Could you check a few things on this model? Use its own coordinates, in mm. A direction names the side the tool comes from. Give positions to 0.01 mm unless a question says otherwise; leave off trailing zeros. Loops run counter-clockwise (first coordinate to the right, second up) from the corner with the lowest first, then second, coordinate; pieces in that order, holes last. Notation, with made-up numbers: (25, -16) -> (37, -16) arc R23 ccw to (37, 18) -> close; hole circle Ø11 at (65.25, 45.25). An arc over 180 degrees is marked (long way). Put each result on its own line as item: value.
```python
from build123d import *

# Parameters (mm, degrees)
F0_R     = 11
F1_DEPTH = 3
F3_DEPTH = 3
F4_R     = 1
F5_DEPTH = 1


with BuildPart() as f1:
    # F0 (on Top) → F1 (new body)
    with BuildSketch(Plane.XY):
        Circle(F0_R)
    extrude(amount=F1_DEPTH)

    # F2 (on face) → F3 (cut)
    with BuildSketch(Plane.XY.offset(3)):
        with BuildLine():
            ThreePointArc((1.140175, -1.05), (0, 1.55), (-1.140175, -1.05))
            Line((-1.140175, -1.05), (1.140175, -1.05))
        make_face()
    extrude(amount=-F3_DEPTH, mode=Mode.SUBTRACT)

    # F4 (on face) → F5 (cut)
    with BuildSketch(Plane.XY.offset(3)):
        with Locations((-1.606246, 9.109472)):
            Circle(F4_R)
        with Locations((-7.085911, -5.945785)):
            Circle(F4_R)
        with Locations((1.606246, 9.109472)):
            Circle(F4_R)
        with Locations((-8.692157, -3.163686)):
            Circle(F4_R)
        with Locations((8.692157, -3.163686)):
            Circle(F4_R)
        with Locations((7.085911, -5.945785)):
            Circle(F4_R)
    extrude(amount=-F5_DEPTH, mode=Mode.SUBTRACT)


solid = f1.part
```
1. If we section it at D-D (y = 9.75): List the corners of the cut face in (x, z) for me, then the cut area to 3 significant figures.
Recorded:
outline: (-5.09, 0) -> (5.09, 0) -> (5.09, 3) -> (2.37, 3) -> (2.37, 2) -> (0.84, 2) -> (0.84, 3) -> (-0.84, 3) -> (-0.84, 2) -> (-2.37, 2) -> (-2.37, 3) -> (-5.09, 3) -> close
area: 27.5 mm^2
2. For faces 1 (the face through (0, -2, 0)), 2 (the face through (0, -1.05, 2)), 3 (the face through (-1.74, 10.1, 2.51)), which set-ups out of +Z, -Z, +X, -X, +Y, -Y let a thin tool reach every point of the face, with its end or its side?
Recorded:
face 1: -Z, +X, -X, +Y, -Y
face 2: +Z, -Z
face 3: +Z
3. I'm going to push flat-ended pins straight in: pin 1 (2 mm diameter, centred on x = -9, y = -3, fed in from +Z); pin 2 (1 mm diameter, centred on x = -8, z = 2.5, fed in from -Y); pin 3 (1.2 mm diameter, centred on x = -7.09, y = -5.95, fed in from +Z). Where does each tip first touch, or does it pass through?
Recorded:
pin 1: stops at z = 3
pin 2: stops at y = -8.05
pin 3: stops at z = 2
4. I need wall thicknesses on line 1 (Y direction, x = 0, z = 1.55); line 2 (Y direction, x = 0.75, z = 2.3); line 3 (X direction, y = 9, z = 2.05). Which ranges of each line are inside material? Lowest first, please.
Recorded:
line 1: y = -11 to -1.05, 1.55 to 11
line 2: y = -10.97 to -1.05, 1.36 to 8.59, 9.63 to 10.97
line 3: x = -6.32 to -2.6, -0.61 to 0.61, 2.6 to 6.32
5. If we section it at C-C (z = 1.5): List the corners of the cut face in (x, y) for me.
Recorded:
outline: circle Ø22 at (0, 0); hole (-1.14, -1.05) -> (1.14, -1.05) arc R1.55 ccw (long way) to start
6. If we section it at B-B (y = 0): List the corners of the cut face in (x, z) for me.
Recorded:
outline: (-11, 0) -> (-1.55, 0) -> (-1.55, 3) -> (-11, 3) -> close; (1.55, 0) -> (11, 0) -> (11, 3) -> (1.55, 3) -> close
7. Thinking about a two-plate mould opening in Y: for faces 4 (the face through (9.646, -2.863, 2.507)), 5 (the face through (-2.38, -10.74, 1.48)), 6 (the face through (0, -2, 3)), which applies, pulls with the +Y half, pulls with the -Y half, needs draft (parallel to the pull), parting line crosses it, or undercut?
Recorded:
face 4: undercut
face 5: parting line crosses it
face 6: needs draft
8. If we section it at A-A (x = 0): List the corners of the cut face in (y, z) for me.
Recorded:
outline: (-11, 0) -> (-1.05, 0) -> (-1.05, 3) -> (-11, 3) -> close; (1.55, 0) -> (11, 0) -> (11, 3) -> (1.55, 3) -> close
